Build history of the part. All positions in model axes, mm. A direction names the side the tool comes from. Round coordinates to 2 decimals unless told otherwise and drop trailing zeros. Write each loop counter-clockwise with the first axis right and the second up, starting at its lowest first coordinate (ties: lowest second). Pieces come first, ordered by that corner, then holes.
1) Which spindle directions (+Z, -Z, +X, -X, +Y, -Y) get a long thin tool onto all of the face, cutting with end or side? Do faces 4 (the cylindrical face through (-2.083, 121.507, 66.864)), 5 (the flat face through (19, 118, 40)), 6 (the cylindrical face through (21.804, 116.513, 45.437)). Say none if no direction does.
2) Saw through at A-A (x = 0). Write the cut outline in (y, z), plus the area to 3 significant figures.
3) Saw through at C-C (x = -22). Write the cut outline in (y, z).
4) Wall check: probe 1 along X at (y, z) = (118, 34.5); probe 2 along Z at (x, y) = (0, 116.5); probe 3 along X at (y, z) = (118, 44.75). Give the ranges that are in metal, low to high.
5) Saw through at B-B (z = 51). Write the cut outline in (x, y).
6) Flat gauge pin, fed straight in: pin 1 (2.5 mm diameter, centred on x = 22, y = 118, fed in from -Z). Where does the tip first touch, or does it go through?
7) Pull direction Y, two halves, no side cores. Call faces 1 (the flat face through (0, 122, 69)), 2 (the flat face through (-22, 118, 50)), 3 (the flat face through (20.6, 117.1, 41)): +Y half, -Y half, draft (parallel to the pull), parting line (faces both ways), or undercut.
8) Saw through at D-D (z = 43.5). Write the cut outline in (x, y), plus the area to 3 significant figures.
from build123d import *

# Parameters (mm, degrees)
TUBE044_R                    = 16
TUBE044_R_2                  = 8.5
TUBE044_DEPTH                = 10
CYLINDER1883_R               = 1.5
CYLINDER1883_DEPTH           = 50
CYLINDER1883_PLACEMENT_ANGLE = 45
CYLINDER1884_R               = 1.5
CYLINDER1884_DEPTH           = 50
CYLINDER1884_PLACEMENT_ANGLE = 45
BOX792_W                     = 8
BOX792_H                     = 6
BOX792_DEPTH                 = 2
BOX793_W                     = 8
BOX793_H                     = 6
BOX793_DEPTH                 = 2
CYLINDER1878_R               = 12
CYLINDER1878_DEPTH           = 20
BOX787_W                     = 56
BOX787_H                     = 8
BOX787_DEPTH                 = 49


with BuildPart() as f_6003_2rs004:
    # Tube044 → Tube044 (new body)
    with BuildSketch(Plane(origin=(0, 131, 51), x_dir=(1, 0, 0), z_dir=(0, -1, 0))):
        Circle(TUBE044_R)
        Circle(TUBE044_R_2, mode=Mode.SUBTRACT)
    extrude(amount=TUBE044_DEPTH)


with BuildPart() as obj1:
    # Cylinder1883 → Cylinder1883 (new body)
    with BuildSketch(Plane.XY):
        Circle(CYLINDER1883_R)
    extrude(amount=CYLINDER1883_DEPTH)


with BuildPart() as obj1_1:
    # Cylinder1883 placement: moved
    add(obj1.part.moved(Location((22, 118, 0))).rotate(Axis((22, 118, 0), (0, 0, 1)), CYLINDER1883_PLACEMENT_ANGLE))


with BuildPart() as compound947:
    # Cylinder1884 → Cylinder1884 (new body)
    with BuildSketch(Plane.XY):
        Circle(CYLINDER1884_R)
    extrude(amount=CYLINDER1884_DEPTH)


with BuildPart() as compound947_1:
    # Cylinder1884 placement: moved
    add(compound947.part.moved(Location((-22, 118, 0))).rotate(Axis((-22, 118, 0), (0, 0, 1)), CYLINDER1884_PLACEMENT_ANGLE))

    # Compound947: union obj1
    add(obj1_1.part)


with BuildPart() as krychle792:
    # Box792 → Box792 (new body)
    with BuildSketch(Plane(origin=(-19, 114, 39), x_dir=(0, 1, 0), z_dir=(0, 0, 1))):
        with Locations((4, 3)):
            Rectangle(BOX792_W, BOX792_H)
    extrude(amount=BOX792_DEPTH)


with BuildPart() as compound946:
    # Box793 → Box793 (new body)
    with BuildSketch(Plane(origin=(25, 114, 39), x_dir=(0, 1, 0), z_dir=(0, 0, 1))):
        with Locations((4, 3)):
            Rectangle(BOX793_W, BOX793_H)
    extrude(amount=BOX793_DEPTH)

    # Compound946: union Krychle792
    add(krychle792.part)


with BuildPart() as obj2:
    # Cylinder1878 → Cylinder1878 (new body)
    with BuildSketch(Plane(origin=(0, 124, 51), x_dir=(1, 0, 0), z_dir=(0, -1, 0))):
        Circle(CYLINDER1878_R)
    extrude(amount=CYLINDER1878_DEPTH)


with BuildPart() as cut598:
    # Box787 → Box787 (new body)
    with BuildSketch(Plane(origin=(-28, 114, 29), x_dir=(1, 0, 0), z_dir=(0, 0, 1))):
        with Locations((28, 4)):
            Rectangle(BOX787_W, BOX787_H)
    extrude(amount=BOX787_DEPTH)

    # Cut591: cut obj2
    add(obj2.part, mode=Mode.SUBTRACT)

    # Cut592: cut Compound946
    add(compound946.part, mode=Mode.SUBTRACT)

    # Cut593: cut Compound947
    add(compound947_1.part, mode=Mode.SUBTRACT)

    # Cut598: cut 6003-2RS004
    add(f_6003_2rs004.part, mode=Mode.SUBTRACT)


solid = cut598.part
Evaluation:
1. face 4: +Y
1. face 5: +Y, -Y
1. face 6: -Z
2. outline: (114, 29) - (122, 29) - (122, 35) - (121, 35) - (121, 39) - (114, 39) - close; (114, 63) - (121, 63) - (121, 67) - (122, 67) - (122, 78) - (114, 78) - close
2. area: 192 mm2
3. outline: (114, 29) - (116.5, 29) - (116.5, 39) - (114, 39) - close; (114, 41) - (116.5, 41) - (116.5, 50) - (119.5, 50) - (119.5, 41) - (122, 41) - (122, 78) - (114, 78) - close; (119.5, 29) - (122, 29) - (122, 39) - (119.5, 39) - close
4. probe 1: x = -28 to -23.5, -20.5 to 20.5, 23.5 to 28
4. probe 2: z = 29 to 39, 63 to 78
4. probe 3: x = -28 to -23.5, -20.5 to -10.24, 10.24 to 20.5, 23.5 to 28
5. outline: (-28, 114) - (-12, 114) - (-12, 121) - (-16, 121) - (-16, 122) - (-28, 122) - close; (12, 114) - (28, 114) - (28, 122) - (16, 122) - (16, 121) - (12, 121) - close
6. pin 1: stops at z = 50
7. face 1: +Y half
7. face 2: undercut
7. face 3: draft
8. outline: (-28, 114) - (-9.37, 114) - (-9.37, 121) - (-14.13, 121) - (-14.13, 122) - (-28, 122) - close; (9.37, 114) - (28, 114) - (28, 122) - (14.13, 122) - (14.13, 121) - (9.37, 121) - close; hole circle Ø3 at (-22, 118); hole circle Ø3 at (22, 118)
8. area: 274 mm2
